```python
from build123d import *

# Parameters (mm, degrees)
SKETCH_1_R      = 500
EXTRUDE_1_DEPTH = 50
SKETCH_2_R      = 25
EXTRUDE_2_DEPTH = 700
SKETCH_3_R      = 25
EXTRUDE_3_DEPTH = 700
SKETCH_4_R      = 25
EXTRUDE_4_DEPTH = 700
SKETCH_5_R      = 25
EXTRUDE_5_DEPTH = 700


with BuildPart() as part:
    # 草图1 → 凸台-拉伸1 (new body)
    with BuildSketch(Plane.XY):
        Circle(SKETCH_1_R)
    extrude(amount=EXTRUDE_1_DEPTH)

    # 草图2 → 凸台-拉伸2 (add)
    with BuildSketch(Plane.XY):
        with Locations((250, 250)):
            Circle(SKETCH_2_R)
    extrude(amount=EXTRUDE_2_DEPTH)

    # 草图3 → 凸台-拉伸3 (add)
    with BuildSketch(Plane.XY):
        with Locations((-250, 250)):
            Circle(SKETCH_3_R)
    extrude(amount=EXTRUDE_3_DEPTH)

    # 草图4 → 凸台-拉伸4 (add)
    with BuildSketch(Plane.XY):
        with Locations((250, -250)):
            Circle(SKETCH_4_R)
    extrude(amount=EXTRUDE_4_DEPTH)

    # 草图5 → 凸台-拉伸5 (add)
    with BuildSketch(Plane.XY):
        with Locations((-250, -250)):
            Circle(SKETCH_5_R)
    extrude(amount=EXTRUDE_5_DEPTH)


solid = part.part
```
Geometry check sheet. Reference: the model listing, model coordinates, mm. A direction names the side the tool comes from. Give positions to 0.01 mm unless a question says otherwise; leave off trailing zeros. Loops run counter-clockwise (first coordinate to the right, second up) from the corner with the lowest first, then second, coordinate; pieces in that order, holes last. Notation, with made-up numbers: M 63,40.25 L 118,40.25 A31 ccw 118,77.25 Z; hole C -38.75,7.5 d3. An arc over 180 degrees is marked long. Write item = value, one per line. Start each with the question number.
1. Section check D-D, the plane y = 0. Enter the section's corners in (x, z).
2. Thickness scan on probe 1 along Z at (x, y) = (146.5, -138.5); probe 2 along X at (y, z) = (-235.5, 305.5); probe 3 along Y at (x, z) = (236, 659). Record the ranges inside material, lowest first.
3. Section check A-A, the plane z = 357.5. Enter the section's corners in (x, y).
4. Draft check along X on faces 1 (the face through (-499.516, 21.984, 24.65)), 2 (the face through (-226.154, 257.509, 370.45)), 3 (the face through (-250, 250, 700)). Enter one of: +X half, -X half, draft (parallel to the pull), parting line (faces both ways), or undercut.
5. Section check B-B, the plane x = 250. Enter the section's corners in (y, z), plus the area to 3 significant figures.
6. Tool access check on faces 4 (the face through (-250, -250, 700)), 5 (the face through (263.44, -228.92, 370.45)). Record the directions out of +Z, -Z, +X, -X, +Y, -Y that give a thin tool (end or side, any length) a straight path to the whole face; none if there is none.
7. Go/stop test with a flat-tipped pin: P1, Ø1, axis at x = -127, y = -395, coming from the +Z side. Record where the tip stops, or that it passes through.
Values follow:
q1.outline = M -500,0 L 500,0 L 500,50 L -500,50 Z
q2.probe_1 = 0 to 50
q2.probe_2 = -270.37 to -229.63, 229.63 to 270.37
q2.probe_3 = -270.71 to -229.29, 229.29 to 270.71
q3.outline = C -250,-250 d50; C -250,250 d50; C 250,-250 d50; C 250,250 d50
q4.face_1 = parting line
q4.face_2 = undercut
q4.face_3 = draft
q5.outline = M -433.01,0 L 433.01,0 L 433.01,50 L 275,50 L 275,700 L 225,700 L 225,50 L -225,50 L -225,700 L -275,700 L -275,50 L -433.01,50 Z
q5.area = 108,000 mm^2
q6.face_4 = +Z, +X, -X, +Y, -Y
q6.face_5 = +Z
q7.P1 = 50
